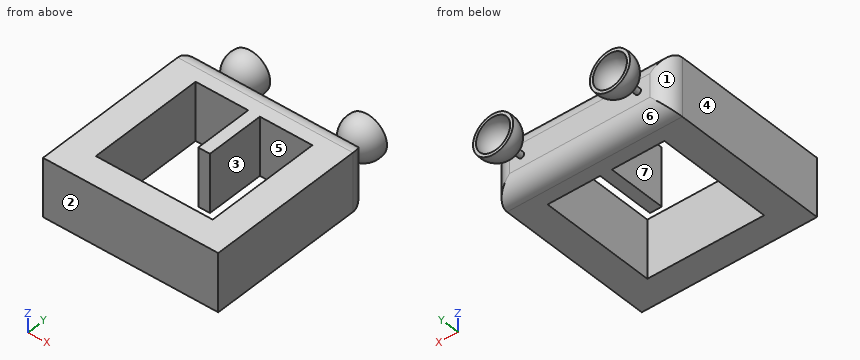
```python
from build123d import *

# Parameters (mm, degrees)
SKETCH1_W           = 30
SKETCH1_H           = 30
BOSS_EXTRUDE1_DEPTH = 10
FILLET1_R           = 3
SKETCH5_W           = 20
SKETCH5_H           = 20
CUT_EXTRUDE1_DEPTH  = 21
SKETCH6_R           = 0.5
BOSS_EXTRUDE4_DEPTH = 2
SKETCH9_W           = 2
SKETCH9_H           = 10
BOSS_EXTRUDE6_DEPTH = 10


with BuildPart() as part:
    # Sketch1 → Boss-Extrude1 (new body)
    with BuildSketch(Plane.XY):
        with Locations((15, 15)):
            Rectangle(SKETCH1_W, SKETCH1_H)
    extrude(amount=BOSS_EXTRUDE1_DEPTH)

    # Fillet1
    fillet1_edges = [part.edges().sort_by_distance(p)[0] for p in [
        (15, 30, 10),
        (15, 30, 0),
        (0, 30, 5),
        (30, 30, 5),
    ]]
    fillet(fillet1_edges, radius=FILLET1_R)

    # Sketch5 → Cut-Extrude1 (cut)
    with BuildSketch(Plane(origin=(0, 0, 0), x_dir=(-1, 0, 0), z_dir=(0, 0, -1))):
        with Locations((-15, 14.738245614)):
            Rectangle(SKETCH5_W, SKETCH5_H)
    extrude(amount=-CUT_EXTRUDE1_DEPTH, mode=Mode.SUBTRACT)

    # Sketch6 → Boss-Extrude4 (add)
    with BuildSketch(Plane(origin=(0, 30, 0), x_dir=(1, 0, 0), z_dir=(0, 1, 0))):
        with Locations(Location((5, -5, 0), (0, 0, 90))):
            Circle(SKETCH6_R)
    boss_extrude4 = extrude(amount=BOSS_EXTRUDE4_DEPTH)

    # Sketch7 → Revolve1 (revolve)
    with BuildSketch(Plane.ZY.offset(-5)):
        with BuildLine():
            Line((5, 32), (5, 31.5))
            ThreePointArc((5, 31.5), (7.698400535, 32.770956583), (8.437058256, 35.660780255))
            Line((8.437058256, 35.660780255), (7.926323539, 35.660780255))
            ThreePointArc((7.926323539, 35.660780255), (7.343324643, 33.126812979), (5, 32))
        make_face()
    revolve1 = revolve(axis=Axis((5, 32, 5), (0, -1, 0)))

    # Mirror3: Boss-Extrude4, Revolve1 across plane
    add(boss_extrude4.mirror(Plane.ZY.offset(-15)))
    add(revolve1.mirror(Plane.ZY.offset(-15)))

    # Sketch9 → Boss-Extrude6 (add)
    with BuildSketch(Plane.XY.offset(10)):
        with Locations((14.994821354, 19.738245614)):
            Rectangle(SKETCH9_W, SKETCH9_H)
    extrude(amount=-BOSS_EXTRUDE6_DEPTH)


solid = part.part
```
The listing builds one solid part. Answer for the finished solid, in the listing's coordinates (mm). Face numbers are marked on the shaded views. A direction names the side the tool comes from. Coordinates: 2 decimals unless noted, no trailing zeros. Loops run counter-clockwise (first coordinate to the right, second up) from the corner with the lowest first, then second, coordinate; pieces in that order, holes last. Notation, with made-up numbers: (55, 77) - (94, 77) arc R21 cw to (94, 99) - close; hole circle Ø7 at (62.5, 16.25). An arc over 180 degrees is marked (long way). Use a Markdown table: item, result. Add a question column.
1) The part is cut by section B-B, the plane y = 13. Give the vertices of the cut face in (x, z), and give its area (3 significant figures).
2) Find the intervals of material crossed by line 1 (X direction, y = 16, z = 9.75); line 2 (Y direction, x = 10.75, z = 7); line 3 (X direction, y = 5.5, z = 1.75), in increasing order.
3) The mould has two halves that part along X. Classify the marked faces 4, 5, 6 and 7: released by +X, released by -X, zero draft, split by the parting line, or undercut.
4) The part is cut by section A-A, the plane x = 21. Give the vertices of the cut face in (y, z), and give its area (3 significant figures).
5) For the marked faces 1, 2 and 3, determine the directions among +Z, -Z, +X, -X, +Y, -Y from which every point of the face is accessible in a straight line to the end or side of a thin tool.
6) Given pin 1 (2 mm diameter, centred on x = 14, z = 5.5, fed in from +Y), flat-ended and moving along its own axis, determine where the tip first touches the part or whether it passes through.
7) The part is cut by section C-C, the plane z = 7.5. Give the vertices of the cut face in (x, y), and give its area (3 significant figures).
8) The part is cut by section D-D, the plane z = 1. Give the vertices of the cut face in (x, y), and give its area (3 significant figures).
Here are the results:
| question | item | result |
|---|---|---|
| 1 | outline | (0, 0) - (5, 0) - (5, 10) - (0, 10) - close; (25, 0) - (30, 0) - (30, 10) - (25, 10) - close |
| 1 | area | 100 mm^2 |
| 2 | line 1 | x = 0 to 5, 13.99 to 15.99, 25 to 30 |
| 2 | line 2 | y = 0 to 4.74, 24.74 to 30 |
| 2 | line 3 | x = 0 to 5, 25 to 30 |
| 3 | face 4 | released by -X |
| 3 | face 5 | undercut |
| 3 | face 6 | zero draft |
| 3 | face 7 | undercut |
| 4 | outline | (0, 0) - (4.74, 0) - (4.74, 10) - (0, 10) - close; (24.74, 0) - (27, 0) arc R3 ccw to (30, 3) - (30, 7) arc R3 ccw to (27, 10) - (24.74, 10) - close |
| 4 | area | 96.1 mm^2 |
| 5 | face 1 | +Z, -Z, -X |
| 5 | face 2 | +Z, -Z, +X, -X, -Y |
| 5 | face 3 | +Z, -Z |
| 6 | pin 1 | stops at y = 30 |
| 7 | outline | (0, 0) - (30, 0) - (30, 27) arc R3 ccw to (27.5, 29.96) - (2.5, 29.96) arc R3 ccw to (0, 27) - close; (2.64, 35.66) arc R2.45 ccw (long way) to (7.36, 35.66) - (6.52, 35.66) arc R1.66 cw (long way) to (3.48, 35.66) - close; (22.64, 35.66) arc R2.45 ccw (long way) to (27.36, 35.66) - (26.52, 35.66) arc R1.66 cw (long way) to (23.48, 35.66) - close; hole (5, 4.74) - (25, 4.74) - (25, 24.74) - (15.99, 24.74) - (15.99, 14.74) - (13.99, 14.74) - (13.99, 24.74) - (5, 24.74) - close |
| 7 | area | 527 mm^2 |
| 8 | outline | (0, 0) - (30, 0) - (30, 27) arc R3 ccw to (29, 29.24) - (1, 29.24) arc R3 ccw to (0, 27) - close; hole (5, 4.74) - (25, 4.74) - (25, 24.74) - (15.99, 24.74) - (15.99, 14.74) - (13.99, 14.74) - (13.99, 24.74) - (5, 24.74) - close |
| 8 | area | 496 mm^2 |
